Read the model definition and answer for the solid it produces. Units are mm, in the model's axes. A direction names the side the tool comes from. Give positions to 0.01 mm unless a question says otherwise; leave off trailing zeros. Loops run counter-clockwise (first coordinate to the right, second up) from the corner with the lowest first, then second, coordinate; pieces in that order, holes last.
(1) Straight lines are drawn through the part: probe 1 along Z at (x, y) = (30, -26) (3 decimals); probe 2 along Y at (x, z) = (42, 34.5); probe 3 along X at (y, z) = (-11.5, -2) (3 decimals). For each, find the intervals that lie inside material, in ascending order.
(2) Find section C-C, the plane x = 98. Write down the section's boundary in (y, z) (3 decimals).
(3) Determine the mould class of faces 5 (the face through (63, 0, 61.925)), 6 (the face through (90, 0, 38.1)), 7 (the face through (22.225, -17, 18)), 8 (the face through (62, 0, 42.875)) for opening direction X: pulls with the +X half, pulls with the -X half, needs draft (parallel to the pull), parting line crosses it, or undercut.
(4) Find section B-B, the plane y = 14.5. Write down the section's boundary in (x, z) (3 decimals), then the cut area to 3 significant figures.
(5) Which of the six approach directions +Z, -Z, +X, -X, +Y, -Y give full straight-line access (tool end or side, diameter ignored) to faces 1 (the face through (5, -7.938, 32)), 2 (the face through (48, -25.4, 42)), 3 (the face through (48, 25.4, 42)), 4 (the face through (32.73, 16.55, 51.97))?
(6) Find section A-A, the plane z = 1. Write down the section's boundary in (x, y) (3 decimals).
(7) Each of these flat-tipped pins is pushed along its axis until it touches: P1, Ø5, axis at y = -18.5, z = 21.5, coming from the -X side (3 decimals); P2, Ø6, axis at y = -4, z = 16.5, coming from the +X side (3 decimals); P3, Ø16, axis at x = 70, y = 3.5, coming from the -Z side. Where does it stop, or does it pass through?
```python
from build123d import *

# Parameters (mm, degrees)
F1_DEPTH = 63.5
F0_W     = 25.3957551599
F0_H     = 19.05
F2_DEPTH = 25.4
F3_DEPTH = 7.9375


with BuildPart() as f1:
    # F0 (on Front) → F1 (new body, symmetric)
    with BuildSketch(Plane.XZ):
        Polygon((-41.275, 9.525), (-41.275, -9.525), (41.275, -9.525), (41.275, 9.525), (22.225, 9.525), align=None)
    extrude(amount=F1_DEPTH, both=True)

    # F0 (on Front) → F2 (join, symmetric)
    with BuildSketch(Plane.XZ):
        with BuildLine():
            Line((22.225, 9.525), (41.275, 9.525))
            Line((41.275, 9.525), (41.275, 27.0002))
            ThreePointArc((41.275, 27.0002), (45.9246798487, 38.2255201513), (57.15, 42.8752))
            Line((57.15, 42.8752), (64.2539668202, 42.8752))
            Line((64.2539668202, 42.8752), (64.2539668202, 61.9252))
            Line((64.2539668202, 61.9252), (57.15, 61.9252))
            ThreePointArc((57.15, 61.9252), (32.4542956671, 51.6959043329), (22.225, 27.0002))
            Line((22.225, 27.0002), (22.225, 9.525))
        make_face()
        with Locations((76.9518444002, 52.4002)):
            Rectangle(F0_W, F0_H)
    extrude(amount=F2_DEPTH, both=True)

    # F0 (on Front) → F3 (join, symmetric)
    with BuildSketch(Plane.XZ):
        with BuildLine():
            add(Edge.make_bspline(
                [(-41.275, 9.525), (-27.2662733646, 37.6478243732), (19.1320432894, 80.2122490874), (57.15, 61.9252)],
                knots=[0, 0, 0, 0, 111.5045361635, 111.5045361635, 111.5045361635, 111.5045361635], degree=3))
            Line((-41.275, 9.525), (22.225, 9.525))
            Line((22.225, 9.525), (22.225, 27.0002))
            ThreePointArc((22.225, 27.0002), (32.4542956671, 51.6959043329), (57.15, 61.9252))
        make_face()
    extrude(amount=F3_DEPTH, both=True)

    # F0 (on Front) → F4 (revolve)
    with BuildSketch(Plane.XZ):
        Polygon((89.6497219801, 66.675), (89.6497219801, 61.9252), (89.6497219801, 42.8752), (89.6497219801, 38.1), (115.0539668202, 38.1), (115.0539668202, 66.675), align=None)
    revolve(axis=Axis((89.6497219801, 0, 52.3875), (0, 0, 1)))


solid = f1.part
```
Entries:
1. probe 1: z = -9.525 to 9.525
1. probe 2: y = -25.4 to 25.4
1. probe 3: x = -41.275 to 41.275
2. outline: (-23.993, 38.1) - (23.993, 38.1) - (23.993, 66.675) - (-23.993, 66.675) - close
3. face 5: undercut
3. face 6: needs draft
3. face 7: pulls with the -X half
3. face 8: undercut
4. outline: (-41.275, -9.525) - (41.275, -9.525) - (41.275, 27) arc R15.875 cw to (57.15, 42.875) - (68.79, 42.875) - (68.79, 38.1) - (110.509, 38.1) - (110.509, 66.675) - (68.79, 66.675) - (68.79, 61.925) - (57.15, 61.925) arc R34.925 ccw to (22.225, 27) - (22.225, 9.525) - (-41.275, 9.525) - close
4. area: 4,080 mm2
5. face 1: +Z, -X, -Y
5. face 2: +Z, +X, -X, -Y
5. face 3: +Z, +X, -X, +Y
5. face 4: +Z, -X, +Y
6. outline: (-41.275, -63.5) - (41.275, -63.5) - (41.275, 63.5) - (-41.275, 63.5) - close
7. P1: stops at x = 22.225
7. P2: stops at x = 41.275
7. P3: stops at z = 38.1
